Could you check a few things on this model? Use its own coordinates, in mm. Face numbers are marked on the shaded views. A direction names the side the tool comes from. Coordinates: 2 decimals unless noted, no trailing zeros. Loops run counter-clockwise (first coordinate to the right, second up) from the corner with the lowest first, then second, coordinate; pieces in that order, holes last. Notation, with made-up numbers: (-13, 52) -> (2, 52) arc R30 ccw to (2, 76) -> close; hole circle Ø11 at (21.5, 37.5). An arc over 180 degrees is marked (long way). One line per question, with ' | ' between items. Start each with the question number.
(1) I'm going to push flat-ended pins straight in: pin 1 Ø5 at (x, y) = (1.5, 11.5) entering from +Z; pin 2 Ø2.5 at (x, z) = (6.75, 6) entering from +Y; pin 3 Ø1.2 at (x, z) = (6.75, -6) entering from +Y; pin 4 Ø8 at (y, z) = (13.5, 20) entering from +X. Where does each tip first touch, or does it pass through?
(2) Suppose I cut it at A-A (z = 4). Please give me the cut outline in (x, y), plus the area to 3 significant figures.
(3) If we mould it in two halves opening along Z, with no side actions, what happens to the marked faces 4, 5 and 6? For each: pulls with the +Z half, pulls with the -Z half, needs draft (parallel to the pull), parting line crosses it, or undercut.
(4) Suppose I cut it at C-C (x = -1.25). Please give me the cut outline in (y, z).
(5) Suppose I cut it at D-D (y = 18). Please give me the cut outline in (x, z).
(6) If I drill on line 1 along X through (y, z) = (1.4, 6); line 2 along Z through (x, y) = (6.75, 0.7); line 3 along Z through (x, y) = (-5, 6.5), over which ranges is the centre line in solid material (lowest first)?
(7) Which directions (+Z, -Z, +X, -X, +Y, -Y) give clear straight access to the entire face, cutting with the end or side of a thin tool? Please do the marked faces 1, 2 and 3.
(8) Suppose I cut it at B-B (z = -6). Please give me the cut outline in (x, y), plus the area to 3 significant figures.
```python
from build123d import *

# Parameters (mm, degrees)
SKETCH_1_R          = 1
EXTRUDE_1_DEPTH     = 3
SKETCH_2_W          = 16.007753667
SKETCH_2_H          = 50
EXTRUDE_2_DEPTH     = 80
CUT_EXTRUDE_1_DEPTH = 89.149011211
CUT_EXTRUDE_2_DEPTH = 81.960252593
EXTRUDE_3_DEPTH     = 3
CUT_EXTRUDE_3_DEPTH = 82.357621032
FILLET_1_R          = 0.5
FILLET_2_R          = 0.2


with BuildPart() as part:
    # 草图1 → 凸台-拉伸1 (new body)
    with BuildSketch(Plane(origin=(0, 0, 0), x_dir=(1, 0, 0), z_dir=(0, 1, 0))):
        with BuildLine():
            Line((-9.25, 25), (7.25, 25))
            ThreePointArc((7.25, 25), (8.664213562, 24.414213562), (9.25, 23))
            Line((9.25, 23), (9.25, -23))
            ThreePointArc((9.25, -23), (8.664213562, -24.414213562), (7.25, -25))
            Line((7.25, -25), (-9.25, -25))
            Line((-9.25, -25), (-9.25, 25))
        make_face()
        with Locations(Location((-1.25, 6, 0), (0, 0, 270))):
            Circle(SKETCH_1_R, mode=Mode.SUBTRACT)
        with Locations(Location((-1.25, -6, 0), (0, 0, 270))):
            Circle(SKETCH_1_R, mode=Mode.SUBTRACT)
        with Locations(Location((6.75, -6, 0), (0, 0, 270))):
            Circle(SKETCH_1_R, mode=Mode.SUBTRACT)
        with Locations(Location((6.75, 6, 0), (0, 0, 270))):
            Circle(SKETCH_1_R, mode=Mode.SUBTRACT)
    extrude(amount=EXTRUDE_1_DEPTH)

    # 草图2 → 凸台-拉伸2 (add)
    with BuildSketch(Plane(origin=(0, 3, 0), x_dir=(1, 0, 0), z_dir=(0, 1, 0))):
        with Locations((-1.246123166, 0)):
            Rectangle(SKETCH_2_W, SKETCH_2_H)
    extrude(amount=EXTRUDE_2_DEPTH)

    # 草图3 → 切除-拉伸1 (cut, through all)
    with BuildSketch(Plane(origin=(6.757753667, 0, 0), x_dir=(0, 0, -1), z_dir=(1, 0, 0))):
        Polygon((0, 47), (-17, 3), (15, 3), (8, 13), align=None)
        Polygon((25, 3), (15, 15.5), (3.181818182, 63), (-1.818181818, 63), (-25, 3), (-37.679958822, 3), (-37.679958822, 88.436899398), (63.328418147, 88.436899398), (63.328418147, 3), align=None)
    extrude(amount=-CUT_EXTRUDE_1_DEPTH, mode=Mode.SUBTRACT)

    # 草图4 → 切除-拉伸2 (cut, through all)
    with BuildSketch(Plane(origin=(0, 0, -25), x_dir=(-1, 0, 0), z_dir=(0, 0, -1))):
        Polygon((-6.757753667, 3), (8.40756476, 64.742116762), (-6.757753667, 64.742116762), align=None)
    extrude(amount=-CUT_EXTRUDE_2_DEPTH, mode=Mode.SUBTRACT)

    # 草图5 → 凸台-拉伸3 (add)
    with BuildSketch(Plane.ZY.offset(9.25)):
        Polygon((-3.181818182, 63), (-15, 15.5), (-25, 3), (-25, 0), (25, 0), (25, 3), (1.818181818, 63), align=None)
        Polygon((0, 47), (-8, 13), (-15, 3), (17, 3), align=None, mode=Mode.SUBTRACT)
    extrude(amount=EXTRUDE_3_DEPTH)

    # 草图6 → 切除-拉伸3 (cut, through all)
    with BuildSketch(Plane(origin=(0, 0, -25), x_dir=(-1, 0, 0), z_dir=(0, 0, -1))):
        Polygon((9.75, 65), (9.75, 45), (6.75, 15.5), (6.75, 0), (15.065136108, 0), (15.065136108, 65), align=None)
    extrude(amount=-CUT_EXTRUDE_3_DEPTH, mode=Mode.SUBTRACT)

    # 圆角1
    # the kernel refuses this fillet: 0.5 mm, written as the material it adds along each edge
    with BuildSketch(Plane(origin=(-6.75, 3, 17), x_dir=(0, 0, -1), z_dir=(1, 0, 0))) as fillet_1_piece_1_section:
        with BuildLine():
            CenterArc((FILLET_1_R * 1.45840694682, FILLET_1_R), FILLET_1_R, 158.875280854, 111.124719146)
            Line((FILLET_1_R * 0.525608812419, FILLET_1_R * 1.3603992792), (0, 0))
            Line((0, 0), (FILLET_1_R * 1.45840694682, 0))
        make_face()
    fillet_1_piece_1 = extrude(amount=15.33076235, mode=Mode.PRIVATE)
    fillet_1_piece_1 = split(fillet_1_piece_1, bisect_by=Plane(origin=(6.334852861, 4.721743663, 16.763347765), z_dir=(-0.9711342799096352, -0.23853345757858446, 0)), keep=Keep.TOP, mode=Mode.PRIVATE)
    add(fillet_1_piece_1)
    with BuildSketch(Plane(origin=(9.158573119, 3, -15), x_dir=(0, 0, 1), z_dir=(-1, 0, 0))) as fillet_1_piece_2_section:
        with BuildLine():
            CenterArc((FILLET_1_R * 1.92065556157, FILLET_1_R), FILLET_1_R, 145.007979801, 124.992020199)
            Line((FILLET_1_R * 1.10142364105, FILLET_1_R * 1.57346234436), (0, 0))
            Line((0, 0), (FILLET_1_R * 1.92065556157, 0))
        make_face()
    fillet_1_piece_2 = extrude(amount=15.908573119, mode=Mode.PRIVATE)
    fillet_1_piece_2 = split(fillet_1_piece_2, bisect_by=Plane(origin=(6.326718063, 4.754862629, -14.622728055), z_dir=(-0.9711342799096352, -0.23853345757858446, 0)), keep=Keep.TOP, mode=Mode.PRIVATE)
    add(fillet_1_piece_2)
    with BuildSketch(Plane(origin=(6.757753667, 3, 16.019874802), x_dir=(1, 0, 0), z_dir=(0, 0, 1))) as fillet_1_piece_3_section:
        with BuildLine():
            CenterArc((FILLET_1_R * 0.784100158108, FILLET_1_R), FILLET_1_R, 193.8, 76.2)
            Line((-FILLET_1_R * 0.187034121801, FILLET_1_R * 0.761466542421), (0, 0))
            Line((0, 0), (FILLET_1_R * 0.784100158108, 0))
        make_face()
    fillet_1_piece_3 = extrude(amount=8.980125198, mode=Mode.PRIVATE)
    fillet_1_piece_3 = split(fillet_1_piece_3, bisect_by=Plane(origin=(6.823760744, 4.428941995, 24.447908775), z_dir=(0, -0.3603992792021625, -0.9327981344055968)), keep=Keep.TOP, mode=Mode.PRIVATE)
    fillet_1_piece_3 = split(fillet_1_piece_3, bisect_by=Plane(origin=(6.823760744, 1.739503793, 17.487009898), z_dir=(0, 0.3603992792021626, 0.9327981344055968)), keep=Keep.TOP, mode=Mode.PRIVATE)
    add(fillet_1_piece_3)
    with BuildSketch(Plane(origin=(6.757753667, 3, -25), x_dir=(1, 0, 0), z_dir=(0, 0, 1))) as fillet_1_piece_4_section:
        with BuildLine():
            CenterArc((FILLET_1_R * 0.784100158108, FILLET_1_R), FILLET_1_R, 193.8, 76.2)
            Line((-FILLET_1_R * 0.187034121801, FILLET_1_R * 0.761466542421), (0, 0))
            Line((0, 0), (FILLET_1_R * 0.784100158108, 0))
        make_face()
    fillet_1_piece_4 = extrude(amount=10.980125198, mode=Mode.PRIVATE)
    fillet_1_piece_4 = split(fillet_1_piece_4, bisect_by=Plane(origin=(6.823819727, 5.521194882, -22.983044095), z_dir=(0, -0.6246950475544241, 0.7808688094430307)), keep=Keep.TOP, mode=Mode.PRIVATE)
    fillet_1_piece_4 = split(fillet_1_piece_4, bisect_by=Plane(origin=(6.823819727, 0.737200979, -16.583959315), z_dir=(0, 0.5734623443633279, -0.819231920519041)), keep=Keep.TOP, mode=Mode.PRIVATE)
    add(fillet_1_piece_4)
    with BuildSketch(Plane(origin=(-6.75, 3, 17), x_dir=(0, 0, -1), z_dir=(1, 0, 0))) as fillet_1_piece_5a_section:
        with BuildLine():
            CenterArc((FILLET_1_R * 1.45840694682, FILLET_1_R), FILLET_1_R, 158.875280854, 111.124719146)
            Line((FILLET_1_R * 0.525608812419, FILLET_1_R * 1.3603992792), (0, 0))
            Line((0, 0), (FILLET_1_R * 1.45840694682, 0))
        make_face()
    fillet_1_piece_5a = extrude(amount=15.33076235, mode=Mode.PRIVATE)
    fillet_1_piece_5a = split(fillet_1_piece_5a, bisect_by=Plane(origin=(6.770254608, 2.949105284, 16.764105763), z_dir=(0.9711342799096352, 0.23853345757858446, 0)), keep=Keep.TOP, mode=Mode.PRIVATE)
    with BuildSketch(Plane(origin=(6.757753667, 3, 16.019874802), x_dir=(1, 0, 0), z_dir=(0, 0, 1))) as fillet_1_piece_5b_section:
        with BuildLine():
            CenterArc((FILLET_1_R * 0.784100158108, FILLET_1_R), FILLET_1_R, 193.8, 76.2)
            Line((-FILLET_1_R * 0.187034121801, FILLET_1_R * 0.761466542421), (0, 0))
            Line((0, 0), (FILLET_1_R * 0.784100158108, 0))
        make_face()
    fillet_1_piece_5b = extrude(amount=8.980125198, mode=Mode.PRIVATE)
    fillet_1_piece_5b = split(fillet_1_piece_5b, bisect_by=Plane(origin=(6.826253209, 3.240744299, 16.906985157), z_dir=(0, -0.3603992792021626, -0.9327981344055968)), keep=Keep.TOP, mode=Mode.PRIVATE)
    fillet_1_piece_5 = fillet_1_piece_5a & fillet_1_piece_5b
    add(fillet_1_piece_5)
    with BuildSketch(Plane(origin=(6.757753667, 3, -25), x_dir=(1, 0, 0), z_dir=(0, 0, 1))) as fillet_1_piece_6a_section:
        with BuildLine():
            CenterArc((FILLET_1_R * 0.784100158108, FILLET_1_R), FILLET_1_R, 193.8, 76.2)
            Line((-FILLET_1_R * 0.187034121801, FILLET_1_R * 0.761466542421), (0, 0))
            Line((0, 0), (FILLET_1_R * 0.784100158108, 0))
        make_face()
    fillet_1_piece_6a = extrude(amount=10.980125198, mode=Mode.PRIVATE)
    fillet_1_piece_6a = split(fillet_1_piece_6a, bisect_by=Plane(origin=(6.828403151, 3.296038352, -14.792773154), z_dir=(0, -0.5734623443633279, 0.819231920519041)), keep=Keep.TOP, mode=Mode.PRIVATE)
    with BuildSketch(Plane(origin=(9.158573119, 3, -15), x_dir=(0, 0, 1), z_dir=(-1, 0, 0))) as fillet_1_piece_6b_section:
        with BuildLine():
            CenterArc((FILLET_1_R * 1.92065556157, FILLET_1_R), FILLET_1_R, 145.007979801, 124.992020199)
            Line((FILLET_1_R * 1.10142364105, FILLET_1_R * 1.57346234436), (0, 0))
            Line((0, 0), (FILLET_1_R * 1.92065556157, 0))
        make_face()
    fillet_1_piece_6b = extrude(amount=15.908573119, mode=Mode.PRIVATE)
    fillet_1_piece_6b = split(fillet_1_piece_6b, bisect_by=Plane(origin=(6.778509417, 2.915497721, -14.622764636), z_dir=(0.9711342799096352, 0.23853345757858446, 0)), keep=Keep.TOP, mode=Mode.PRIVATE)
    fillet_1_piece_6 = fillet_1_piece_6a & fillet_1_piece_6b
    add(fillet_1_piece_6)

    # 圆角2
    fillet_2_edges = [part.edges().sort_by_distance(p)[0] for p in [
        (-6.899841453, 47, 0),
    ]]
    fillet(fillet_2_edges, radius=FILLET_2_R)


solid = part.part
```
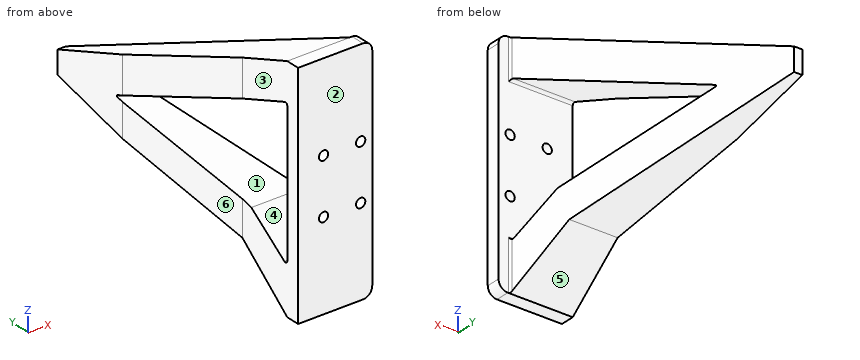
Checks:
1) pin 1: stops at z = 22.68 | pin 2: stops at y = 3 | pin 3: passes through | pin 4: stops at x = 5.16
2) outline: (-9.75, 45) -> (-8.9, 36.65) -> (-1.51, 36.65) -> (-6.59, 57.35) -> (-9.75, 57.35) -> close; (-6.75, 0) -> (9.25, 0) -> (9.25, 3) -> (-6.75, 3) -> close | area: 162 mm^2
3) face 4: undercut | face 5: pulls with the -Z half | face 6: needs draft
4) outline: (0, -25) -> (3, -25) -> (15.5, -15) -> (35.6, -10) -> (35.6, -2.68) -> (13, -8) -> (3.79, -14.45) arc R0.5 cw to (3, -14.04) -> (3, -7) -> (0, -7) -> close; (0, -5) -> (3, -5) -> (3, 5) -> (0, 5) -> close; (0, 7) -> (3, 7) -> (3, 16.27) arc R0.5 cw to (3.68, 16.74) -> (35.6, 4.4) -> (35.6, 12.4) -> (3, 25) -> (0, 25) -> close
5) outline: (-7, -14.38) -> (3.07, -14.38) -> (3.07, -6.82) -> (-7, -6.82) -> close; (-7, 11.2) -> (3.07, 11.2) -> (3.07, 19.2) -> (-7, 19.2) -> close
6) line 1: x = -6.75 to -2.25, -0.25 to 5.75, 7.75 to 9.25 | line 2: z = -25 to -7, -5 to 5, 7 to 25 | line 3: z = -22.2 to -12.55, 15.65 to 23.65
7) face 1: +X, -X | face 2: +Z, -Z, +X, -X, -Y | face 3: +Z, -Z, -X, -Y
8) outline: (-9.75, 45) -> (-7.36, 21.5) -> (2.21, 21.5) -> (-5.2, 51.67) -> (-9.75, 51.67) -> close; (-6.75, 0) -> (-2.25, 0) -> (-2.25, 3) -> (-6.75, 3) -> close; (-0.25, 0) -> (5.75, 0) -> (5.75, 3) -> (-0.25, 3) -> close; (7.75, 0) -> (9.25, 0) -> (9.25, 3) -> (7.75, 3) -> close | area: 257 mm^2
